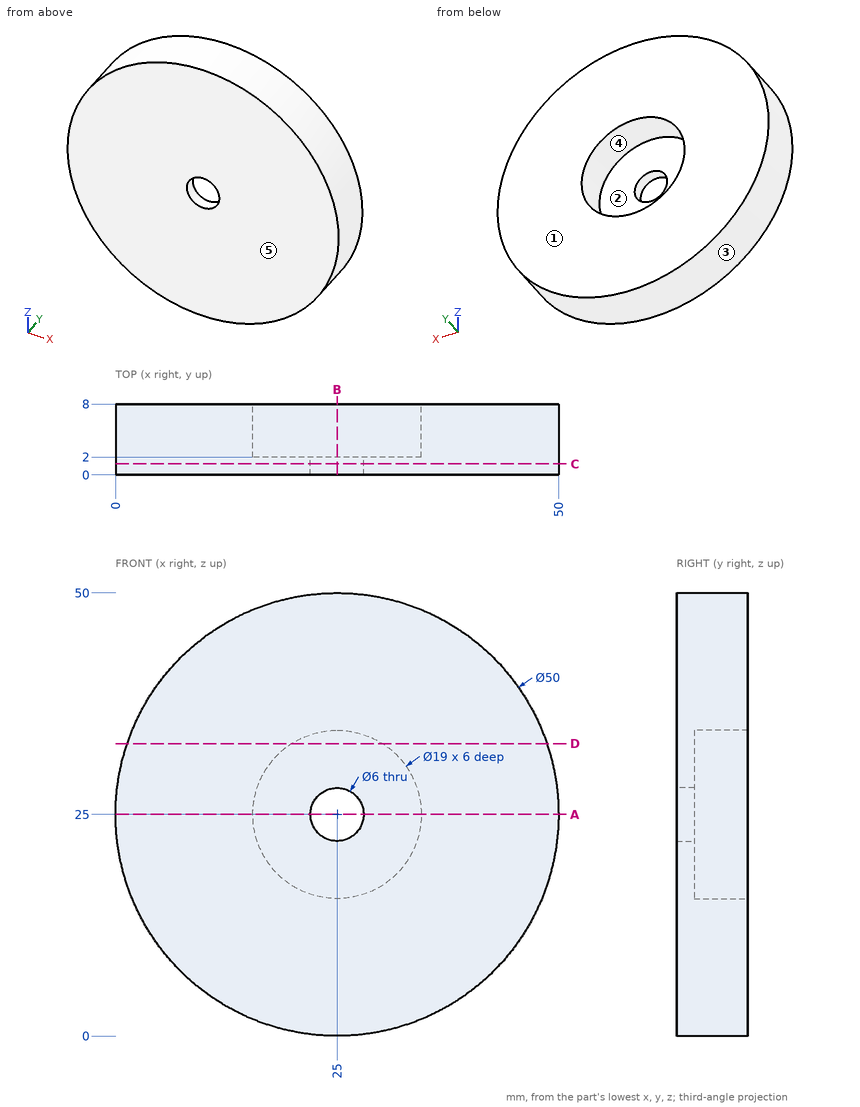
Study the drawing (mm; zero at the part's minimum x, y, z) and answer. A direction names the side the tool comes from. Coordinates: 2 decimals unless noted, no trailing zeros. Loops run counter-clockwise (first coordinate to the right, second up) from the corner with the lowest first, then second, coordinate; pieces in that order, holes last. Notation, with made-up numbers: M 24.25,-32.5 L 80.25,-32.5 A23 cw 80.25,-1.5 Z; hole C 65,16.25 d1. An arc over 180 degrees is marked long. Answer in a Markdown table with one row per item.
1) Given pin 1 (17 mm diameter, centred on x = 25, z = 25, fed in from +Y); pin 2 (4 mm diameter, centred on x = 41.5, y = 3, fed in from -Z); pin 3 (2 mm diameter, centred on x = 34.5, y = 2.5, fed in from +Z), each flat-ended and moving along its own axis, determine where each tip first touches the part or whether it passes through.
Answers below:
| item | result |
|---|---|
| pin 1 | y = 2 |
| pin 2 | z = 4.63 |
| pin 3 | z = 48.51 |
2) Find section B-B (x = 25). Determine the outline of the cut face in (y, z), then the cut area to 3 significant figures.
Answers below:
| item | result |
|---|---|
| outline | M 0,0 L 8,0 L 8,15.5 L 2,15.5 L 2,22 L 0,22 Z; M 0,28 L 2,28 L 2,34.5 L 8,34.5 L 8,50 L 0,50 Z |
| area | 274 mm^2 |
3) Which of the six approach directions +Z, -Z, +X, -X, +Y, -Y give full straight-line access (tool end or side, diameter ignored) to the marked faces 4 and 5?
Answers below:
| item | result |
|---|---|
| face 4 | +Y |
| face 5 | +Z, -Z, +X, -X, -Y |
4) Find section C-C (y = 1.25). Determine the outline of the cut face in (x, z), then the cut area to 3 significant figures.
Answers below:
| item | result |
|---|---|
| outline | C 25,25 d50; hole C 25,25 d6 |
| area | 1,940 mm^2 |
5) Find section A-A (z = 25). Determine the outline of the cut face in (x, y).
Answers below:
| item | result |
|---|---|
| outline | M 0,0 L 22,0 L 22,2 L 15.5,2 L 15.5,8 L 0,8 Z; M 28,0 L 50,0 L 50,8 L 34.5,8 L 34.5,2 L 28,2 Z |
6) Find the intervals of material crossed by probe 1 along X at (y, z) = (4.05, 25); probe 2 along Z at (x, y) = (24.5, 3) (3 decimals); probe 3 along X at (y, z) = (0.5, 25), in increasing order.
Answers below:
| item | result |
|---|---|
| probe 1 | 0 to 15.5, 34.5 to 50 |
| probe 2 | 0.005 to 15.513, 34.487 to 49.995 |
| probe 3 | 0 to 22, 28 to 50 |
7) Find section D-D (z = 33). Determine the outline of the cut face in (x, y), then the cut area to 3 significant figures.
Answers below:
| item | result |
|---|---|
| outline | M 1.31,0 L 48.69,0 L 48.69,8 L 30.12,8 L 30.12,2 L 19.88,2 L 19.88,8 L 1.31,8 Z |
| area | 317 mm^2 |
8) Determine the mould class of the marked faces 1, 2 and 3 for opening direction X: released by +X, released by -X, zero draft, split by the parting line, or undercut.
Answers below:
| item | result |
|---|---|
| face 1 | zero draft |
| face 2 | undercut |
| face 3 | split by the parting line |
